```python
from build123d import *

# Parameters (mm, degrees)
SKETCH1_W               = 40
SKETCH1_H               = 50
BOSS_EXTRUDE1_DEPTH     = 40
CHAMFER1_SIZE           = 10
CHAMFER2_SIZE           = 12
CHAMFER4_SIZE           = 5
BOSS_EXTRUDE2_DEPTH     = 4
CHAMFER5_SIZE           = 2
SHELL1_T                = -2
SKETCH3_W               = 45
SKETCH3_H               = 43
CUT_EXTRUDE1_DEPTH      = 20
CUT_EXTRUDE2_DEPTH      = 69.585712798
CUT_EXTRUDE2_DEPTH_BACK = 10
SKETCH4_R               = 2.5
BOSS_EXTRUDE3_DEPTH     = 2


with BuildPart() as part:
    # Sketch1 → Boss-Extrude1 (new body)
    with BuildSketch(Plane.XY):
        Rectangle(SKETCH1_W, SKETCH1_H)
    extrude(amount=BOSS_EXTRUDE1_DEPTH)

    # Chamfer1
    chamfer1_edges = [part.edges().sort_by_distance(p)[0] for p in [
        (-20, 0, 40),
        (20, 0, 40),
    ]]
    chamfer(chamfer1_edges, length=CHAMFER1_SIZE)

    # Chamfer2
    chamfer2_edges = [part.edges().sort_by_distance(p)[0] for p in [
        (-20, 0, 0),
        (20, 0, 0),
    ]]
    chamfer(chamfer2_edges, length=CHAMFER2_SIZE)

    # Chamfer4
    chamfer4_edges = [part.edges().sort_by_distance(p)[0] for p in [
        (0, -25, 40),
        (20, -25, 21),
        (-20, -25, 21),
        (15, -25, 35),
        (-15, -25, 35),
        (0, -25, 0),
        (14, -25, 6),
        (-14, -25, 6),
    ]]
    chamfer(chamfer4_edges, length=CHAMFER4_SIZE)

    # Sketch2 → Boss-Extrude2 (add)
    with BuildSketch(Plane.XZ.offset(25)):
        Polygon((6.272077939, 31), (-6.272077939, 31), (-11, 26.272077939), (-11, 15.727922061), (-4.272077939, 9), (4.272077939, 9), (11, 15.727922061), (11, 26.272077939), align=None)
    extrude(amount=BOSS_EXTRUDE2_DEPTH)

    # Chamfer5
    chamfer5_edges = [part.edges().sort_by_distance(p)[0] for p in [
        (8.636038969, -29, 28.636038969),
        (0, -29, 31),
        (-8.636038969, -29, 28.636038969),
        (-11, -29, 21),
        (-7.636038969, -29, 12.363961031),
        (0, -29, 9),
        (7.636038969, -29, 12.363961031),
        (11, -29, 21),
    ]]
    chamfer(chamfer5_edges, length=CHAMFER5_SIZE)

    # Shell1
    shell1_openings = [part.faces().sort_by_distance(p)[0] for p in [
        (0, 2.5, 0),
    ]]
    offset(amount=SHELL1_T, openings=shell1_openings, kind=Kind.INTERSECTION)

    # Sketch3 → Cut-Extrude1 (cut)
    with BuildSketch(Plane(origin=(0, 0, 0), x_dir=(-1, 0, 0), z_dir=(0, 0, -1))):
        with Locations((-2.5, 1.5)):
            Rectangle(SKETCH3_W, SKETCH3_H)
    extrude(amount=-CUT_EXTRUDE1_DEPTH, mode=Mode.SUBTRACT)

    # Sketch4 → Cut-Extrude2 (cut, two sides: drawn at the far end of the back side and taken through both)
    with BuildSketch(Plane.XZ.offset(-23).offset(-CUT_EXTRUDE2_DEPTH_BACK)):
        with Locations(Location((-1.222653688, 5.030872217, 0), (0, 0, 161.396212333))):
            Circle(SKETCH4_R)
    extrude(amount=CUT_EXTRUDE2_DEPTH + CUT_EXTRUDE2_DEPTH_BACK, mode=Mode.SUBTRACT)

    # Sketch5 → Boss-Extrude3 (add)
    # profile 1 of 8: a face of its own
    with BuildSketch(Plane.XZ.offset(29)):
        Polygon((-3.907968564, 25.873424225), (-1.8521612, 26.578618027), (2.162403013, 26.578618027), (4.206288315, 25.839581431), (4.183149683, 24.513463944), (0.17410729, 21.92507617), (-3.70376403, 24.56651521), align=None)
        Polygon((-1.267927635, 24.828885337), (1.687291293, 24.828885337), (1.687291293, 24.58450637), (0.167260904, 23.603117877), (-1.267927635, 24.580706539), align=None, mode=Mode.SUBTRACT)
    # profile 2 of 8: a face of its own
    with BuildSketch(Plane.XZ.offset(29)):
        Polygon((-6.640454007, 25.873424225), (-4.222410504, 25.873424225), (-3.990642578, 24.390109498), (-1.452911939, 22.661516611), (-1.008516208, 19.817383934), (-3.786282946, 20.257943712), (-5.746633086, 21.646373557), align=None)
        Polygon((-5.179729537, 24.26393897), (-5.179729537, 23.810064286), (-2.37123808, 21.924837325), (-2.37123808, 22.426829117), align=None, mode=Mode.SUBTRACT)
        Polygon((-4.974230162, 23.056566578), (-4.974230162, 22.684710567), (-2.175342033, 20.805929932), (-2.175342033, 21.167929466), align=None, mode=Mode.SUBTRACT)
    # profile 3 of 8: a face of its own
    with BuildSketch(Plane.XZ.offset(29)):
        Polygon((0.175518811, 21.579113739), (-1.194872838, 22.512565549), (-0.754201781, 19.692270785), (-0.754201781, 16.336897736), (1.148015733, 16.336897736), (1.148015733, 19.6551114), (1.568514987, 22.478484191), align=None)
    # profile 4 of 8: a face of its own
    with BuildSketch(Plane.XZ.offset(29)):
        Polygon((-5.371925401, 21.102931741), (-5.040352094, 15.872748244), (-2.918674263, 14.004045062), (-2.918674263, 18.883324606), (-3.897566255, 19.36360058), (-3.897566255, 20.051937661), align=None)
    # profile 5 of 8: a face of its own
    with BuildSketch(Plane.XZ.offset(29)):
        Polygon((-2.57777667, 18.638279212), (-2.57777667, 13.829972979), (-1.787898039, 13.134274183), (-0.948144856, 15.171513794), (1.44618133, 15.171513794), (2.140445472, 13.131762403), (2.958479742, 13.727080014), (2.958479742, 18.581830676), (1.348015733, 19.245666323), (1.348015733, 16.136897736), (-0.954201781, 16.136897736), (-0.954201781, 19.321874117), align=None)
    # profile 6 of 8: a face of its own
    with BuildSketch(Plane.XZ.offset(29)):
        Polygon((-1.452207759, 13.131762403), (1.872175521, 13.131762403), (1.225826325, 14.867356635), (-0.822603437, 14.867356635), align=None)
    # profile 7 of 8: a face of its own
    with BuildSketch(Plane.XZ.offset(29)):
        Polygon((4.147969201, 20.290315345), (6.096924719, 21.694695099), (6.956223847, 25.928898472), (4.538260846, 25.909167636), (4.318604239, 24.424011104), (1.795063119, 22.674768301), (1.373889836, 19.827104116), align=None)
        Polygon((2.719369869, 21.945606931), (2.715273698, 22.447582011), (5.508681142, 24.307547529), (5.512384685, 23.853687956), align=None, mode=Mode.SUBTRACT)
        Polygon((2.532610443, 20.825138309), (2.529656587, 21.187125792), (5.313040568, 23.098538493), (5.316074852, 22.726694861), align=None, mode=Mode.SUBTRACT)
    # profile 8 of 8: a face of its own
    with BuildSketch(Plane.XZ.offset(29)):
        Polygon((4.266546498, 19.396910041), (4.260929781, 20.085224205), (5.726663904, 21.148213823), (5.43777907, 15.915498866), (3.331420184, 14.029545356), (3.291606068, 18.908662459), align=None)
    extrude(amount=BOSS_EXTRUDE3_DEPTH)


solid = part.part
```
Source: CAD feature listing. Evaluate the final solid. Frame: model axes, mm. A direction names the side the tool comes from. Round coordinates to 2 decimals unless told otherwise and drop trailing zeros. Loops run counter-clockwise (first coordinate to the right, second up) from the corner with the lowest first, then second, coordinate; pieces in that order, holes last. Notation, with made-up numbers: M 40.25,17.5 L 62.25,17.5 A17 cw 62.25,32.5 Z; hole C 19,-33.5 d1. An arc over 180 degrees is marked long. Use a Markdown table: item, result. Add a question column.
1. Cut plane A-A, the plane y = 9.5. Output: boundary loops of the cut face in (x, z), and give its area (3 significant figures).
2. Contact query for flat-ended pins moving along their axis: pin 1 (3 mm diameter, centred on x = -18.5, y = -4, fed in from -Z); pin 2 (1 mm diameter, centred on x = 6, z = 7, fed in from -Y); pin 3 (2 mm diameter, centred on y = -29.5, z = 18, fed in from -X). Output: stop coordinate, or through.
3. Set-up query: faces 1 (the flat face through (-2.894, -29.986, 26.221)), 2 (the flat face through (-13.52, 1.62, 33.65)), 3 (the flat face through (10.88, -21.48, 8.97)), 4 (the flat face through (-6.187, -29.986, 23.73)). Return all of +Z, -Z, +X, -X, +Y, -Y with unobstructed straight access to the full face (end or side cutting, diameter ignored); none if empty.
4. Cut plane C-C, the plane y = -22. Output: boundary loops of the cut face in (x, z), and give its area (3 significant figures).
5. Cut plane D-D, the plane x = -12.5. Output: boundary loops of the cut face in (y, z).
6. Ray query, line 1 along X through (y, z) = (5.5, 28.5); line 2 along Y through (x, z) = (0, 15.5); line 3 along Y through (x, z) = (-3.5, 14). Return the intervals inside material, ascending. Write a range as [from, to].
7. Pull-direction query (Z, two-part tool) for faces 5 (the flat face through (15, 2, 35)), 6 (the flat face through (4.135, -29.986, 22.913)), 7 (the flat face through (-2.919, -30, 16)); classes: +Z half, -Z half, draft (parallel to the pull), parting line (faces both ways), or undercut.
8. Cut plane B-B, the plane z = 33.5. Output: boundary loops of the cut face in (x, y).
Solution:
| question | item | result |
|---|---|---|
| 1 | outline | M -20,20 L -18,20 L -18,29.17 L -9.17,38 L 9.17,38 L 18,29.17 L 18,20 L 20,20 L 20,30 L 10,40 L -10,40 L -20,30 Z |
| 1 | area | 130 mm2 |
| 2 | pin 1 | stops at z = 20 |
| 2 | pin 2 | stops at y = -25 |
| 2 | pin 3 | stops at x = -9.5 |
| 3 | face 1 | +Z, -X, -Y |
| 3 | face 2 | -Z |
| 3 | face 3 | none |
| 3 | face 4 | -Z, -X, -Y |
| 4 | outline | M -18,12.83 L -7.17,2 L 7.17,2 L 18,12.83 L 18,29.17 L 9.17,38 L -9.17,38 L -18,29.17 Z; hole M -15.17,14 L -6,4.83 L -3.71,4.83 A2.5 ccw 1.27,4.83 L 6,4.83 L 15.17,14 L 15.17,28 L 8,35.17 L -8,35.17 L -15.17,28 Z |
| 4 | area | 307 mm2 |
| 5 | outline | M -25,11.57 L -20,4.5 L -20,8.5 L -23,12.74 L -23,29.26 L -19.17,34.67 L 23,34.67 L 23,4.5 L 25,4.5 L 25,37.5 L -20,37.5 L -25,30.43 Z |
| 6 | line 1 | x = [-20, -18], [18, 20] |
| 6 | line 2 | y = [-31, -27], [23, 25] |
| 6 | line 3 | y = [-29, -27], [23, 25] |
| 7 | face 5 | +Z half |
| 7 | face 6 | undercut |
| 7 | face 7 | draft |
| 8 | outline | M -16.5,-20 L -9.43,-25 L 9.43,-25 L 16.5,-20 L 16.5,25 L -16.5,25 Z; hole M -13.67,-19.17 L -8.26,-23 L 8.26,-23 L 13.67,-19.17 L 13.67,23 L -13.67,23 Z |
